Source: CAD feature listing. Evaluate the final solid. Frame: model axes, mm. Face numbers are marked on the shaded views. Give positions to 0.01 mm unless a question says otherwise; leave off trailing zeros. Order: outer loops, then holes, each group sorted by start corner. A loop starts at its lowest first (then second) coordinate and runs counter-clockwise, first axis right, second up.
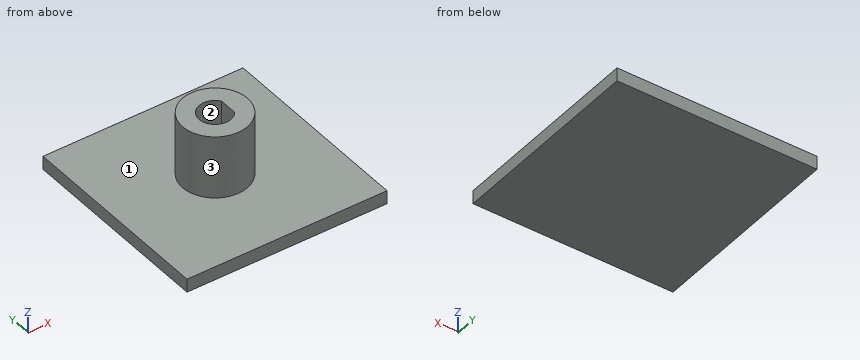
Autodesk Inventor part; units mm, degrees
ref_plane "YZ Plane" through (0, 0, 0) normal (1, 0, 0) x (0, 1, 0)
ref_plane "XZ Plane" through (0, 0, 0) normal (0, 1, 0) x (-1, 0, 0)
ref_plane "XY Plane" through (0, 0, 0) normal (0, 0, 1) x (1, 0, 0)
sketch "Sketch1" plane through (0, 0, 0) normal (0, 0, 1) x (1, 0, 0)
  line L0 (19.05, -19.05) -> (-19.05, -19.05)
  line L1 (-19.05, -19.05) -> (-19.05, 19.05)
  line L2 (-19.05, 19.05) -> (19.05, 19.05)
  line L3 (19.05, 19.05) -> (19.05, -19.05)
  line L4 (19.05, -19.05) -> (-19.05, 19.05) construction
  line L5 (-19.05, -19.05) -> (19.05, 19.05) construction
  point P0 (0, 0)
  dimension "d0" = 38.1
  dimension "d1" = 38.1
extrude "Extrusion1" add sketch "Sketch1" along normal blind 2.54
sketch "Sketch2" plane through (0, 0, 2.54) normal (0, 0, 1) x (1, 0, 0)
  circle A0 centre (0, 0) radius 6.1658
  dimension "d4" = 12.3317
extrude "Extrusion2" add sketch "Sketch2" along normal blind 11.9634
sketch "Sketch3" plane through (0, 0, 14.5034) normal (0, 0, 1) x (1, 0, 0)
  circle A0 centre (0, 0) radius 3.0226
  line L0 (2.4892, 1.7146) -> (2.4892, -1.7146)
  dimension "d7" = 6.0452
  dimension "d8" = 5.5118
extrude "Extrusion3" cut sketch "Sketch3" against normal blind 11.9634 contours L0 A0 picked at (0.6593, -0.1215)
properties part number "Hub Prototype"
1) Section query C-C on z = 4.25. Output: boundary loops of the cut face in (x, y), and give its area (3 significant figures).
Checks:
outline: circle Ø12.33 at (0, 0); hole (2.49, -1.71) - (2.49, 1.71) arc R3.02 ccw (long way) to start
area: 92.0 mm2
2) First-contact query: pin 1 Ø1.5 at (x, z) = (-3.5, 12.5) entering from -Y; pin 2 Ø4 at (y, z) = (0, 7) entering from -X; pin 3 Ø6 at (y, z) = (-10.5, 7.5) entering from -X; pin 4 Ø6 at (x, z) = (-1, 6.5) entering from +Y. Flat tips, straight axial feed; report the tip coordinate or a pass-through.
Checks:
pin 1: stops at y = -5.52
pin 2: stops at x = -6.17
pin 3: passes through
pin 4: stops at y = 6.17
3) Section query B-B on y = 0. Output: boundary loops of the cut face in (x, z), and give its area (3 significant figures).
Checks:
outline: (-19.05, 0) - (19.05, 0) - (19.05, 2.54) - (6.17, 2.54) - (6.17, 14.5) - (2.49, 14.5) - (2.49, 2.54) - (-3.02, 2.54) - (-3.02, 14.5) - (-6.17, 14.5) - (-6.17, 2.54) - (-19.05, 2.54) - close
area: 178 mm2
4) Section query D-D on x = 16. Output: boundary loops of the cut face in (y, z), and give its area (3 significant figures).
Checks:
outline: (-19.05, 0) - (19.05, 0) - (19.05, 2.54) - (-19.05, 2.54) - close
area: 96.8 mm2
5) Section query A-A on x = 0. Output: boundary loops of the cut face in (y, z).
Checks:
outline: (-19.05, 0) - (19.05, 0) - (19.05, 2.54) - (6.17, 2.54) - (6.17, 14.5) - (3.02, 14.5) - (3.02, 2.54) - (-3.02, 2.54) - (-3.02, 14.5) - (-6.17, 14.5) - (-6.17, 2.54) - (-19.05, 2.54) - close
6) Pull-direction query (X, two-part tool) for the marked faces 1, 2 and 3; classes: +X half, -X half, draft (parallel to the pull), parting line (faces both ways), or undercut.
Checks:
face 1: draft
face 2: undercut
face 3: parting line
7) Ray query, L1, parallel to Y at x = 0, z = 9.25; L2, parallel to Z at x = -17, y = -13.5; L3, parallel to Y at x = 1.5, z = 10.75. Return the intervals inside material, ascending.
Checks:
L1: y = -6.17 to -3.02, 3.02 to 6.17
L2: z = 0 to 2.54
L3: y = -5.98 to -2.62, 2.62 to 5.98
